```python
from build123d import *

# Parameters (mm, degrees)
F0_R      = 63.7442234454
F1_DEPTH  = 12.7
F2_R      = 25.4
F3_DEPTH  = 19.05
F4_R      = 9.525
F5_DEPTH  = 50.8
F6_DEPTH  = 12.7
F7_R      = 38.1
F8_DEPTH  = 12.7
F9_W      = 25.4
F9_H      = 25.4
F10_DEPTH = 25.4


with BuildPart() as f1:
    # F0 (on Top) → F1 (new body)
    with BuildSketch(Plane.XY):
        Circle(F0_R)
    extrude(amount=F1_DEPTH)

    # F2 (on face) → F3 (join)
    with BuildSketch(Plane.XY.offset(12.7)):
        Circle(F2_R)
    extrude(amount=F3_DEPTH)

    # F4 (on face) → F5 (cut)
    with BuildSketch(Plane.XY.offset(31.75)):
        Circle(F4_R)
    extrude(amount=-F5_DEPTH, mode=Mode.SUBTRACT)

    # F6 (add): a face of the model
    f6_faces = [f1.faces().sort_by_distance(p)[0] for p in [
        (-24.6815795103, 0, 31.75),
    ]]
    extrude(f6_faces, amount=F6_DEPTH)

    # F7 (on face) → F8 (join)
    with BuildSketch(Plane.XY.offset(44.45)):
        Circle(F7_R)
    extrude(amount=F8_DEPTH)

    # F9 (on face) → F10 (cut)
    with BuildSketch(Plane.XY.offset(57.15)):
        Rectangle(F9_W, F9_H)
    extrude(amount=-F10_DEPTH, mode=Mode.SUBTRACT)


solid = f1.part
```
Model file for the job. Use its own axes, mm. A direction names the side the tool comes from. Give positions to 0.01 mm unless a question says otherwise; leave off trailing zeros. Write each loop counter-clockwise with the first axis right and the second up, starting at its lowest first coordinate (ties: lowest second). Pieces come first, ordered by that corner, then holes. Notation, with made-up numbers: M 33,-39.5 L 77,-39.5 A22 ccw 77,-7.5 Z; hole C 77,85.25 d9. An arc over 180 degrees is marked long. Use a Markdown table: item, result.
1) Cut at C-C (z = 9). List the corners of the cut face in (x, y) (3 decimals), and give its area (3 significant figures).
Responses:
| item | result |
|---|---|
| outline | C 0,0 d127.488; hole C 0,0 d19.05 |
| area | 12,500 mm2 |
2) Pin check, flat tips, straight feed: pin 1 (5 mm diameter, centred on x = 30.5, y = -47, fed in from +Z); pin 2 (20.5 mm diameter, centred on x = 6, z = 47, fed in from -Y); pin 3 (1 mm diameter, centred on y = -13.5, z = 30.5, fed in from +X). Stop position of each tip, or through.
Responses:
| item | result |
|---|---|
| pin 1 | stops at z = 12.7 |
| pin 2 | stops at y = -38.1 |
| pin 3 | stops at x = 21.82 |
3) Cut at A-A (y = 0). List the corners of the cut face in (x, z) (3 decimals).
Responses:
| item | result |
|---|---|
| outline | M -63.744,0 L -9.525,0 L -9.525,31.75 L -12.7,31.75 L -12.7,57.15 L -38.1,57.15 L -38.1,44.45 L -25.4,44.45 L -25.4,12.7 L -63.744,12.7 Z; M 9.525,0 L 63.744,0 L 63.744,12.7 L 25.4,12.7 L 25.4,44.45 L 38.1,44.45 L 38.1,57.15 L 12.7,57.15 L 12.7,31.75 L 9.525,31.75 Z |
4) Drill centre lines: line 1 (Z direction, x = -23, y = -15); line 2 (Y direction, x = 0, z = 21) (3 decimals); line 3 (Z direction, x = 15.5, y = -47). Where is each one in solid material? Low to high. Write a range as from..to.
Responses:
| item | result |
|---|---|
| line 1 | z = 0..12.7, 44.45..57.15 |
| line 2 | y = -25.4..-9.525, 9.525..25.4 |
| line 3 | z = 0..12.7 |
5) Cut at D-D (x = -35.5). List the corners of the cut face in (y, z), and give its area (3 significant figures).
Responses:
| item | result |
|---|---|
| outline | M -52.94,0 L 52.94,0 L 52.94,12.7 L -52.94,12.7 Z; M -13.83,44.45 L 13.83,44.45 L 13.83,57.15 L -13.83,57.15 Z |
| area | 1,700 mm2 |
6) Pull direction X, two halves, no side cores. Call faces 4 (the flat face through (27, 1, 12.7)), 5 (the cylindrical face through (-8.3, 63.2, 6.3)), 6 (the flat face through (0, 12.7, 45)): +X half, -X half, draft (parallel to the pull), parting line (faces both ways), or undercut.
Responses:
| item | result |
|---|---|
| face 4 | draft |
| face 5 | parting line |
| face 6 | undercut |
7) Tool access for faces 1 (the cylindrical face through (-7.559, -5.796, 16.097)), 2 (the flat face through (-12.7, 0, 45)), 3 (the cylindrical face through (-5.506, -24.796, 28.353)): list every direction of +Z, -Z, +X, -X, +Y, -Y with a clear straight run to the whole face (end or side of a thin tool).
Responses:
| item | result |
|---|---|
| face 1 | +Z, -Z |
| face 2 | +Z |
| face 3 | none |
